from build123d import *

# Parameters (mm, degrees)
SKETCH1_W                                  = 43
SKETCH1_H                                  = 43
SKETCH1_R                                  = 1
BOSS_EXTRUDE1_DEPTH                        = 3.5
SKETCH3_R                                  = 1.45
BOSS_EXTRUDE2_DEPTH                        = 5
MIRROR2_AT_THE_SECOND_PLANE_COPY_1_SKETC_R = 1.45
MIRROR2_AT_THE_SECOND_PLANE_COPY_1_DEPTH   = 5
SKETCH4_W                                  = 4.5
SKETCH4_H                                  = 43
BOSS_EXTRUDE3_DEPTH                        = 5.03


with BuildPart() as part:
    # Sketch1 → Boss-Extrude1 (new body)
    with BuildSketch(Plane(origin=(0, 0, 0), x_dir=(1, 0, 0), z_dir=(0, 1, 0))):
        Rectangle(SKETCH1_W, SKETCH1_H)
        with Locations(Location((0, 0, 0), (0, 0, 270))):
            Circle(SKETCH1_R, mode=Mode.SUBTRACT)
    extrude(amount=BOSS_EXTRUDE1_DEPTH)

    # Sketch3 → Boss-Extrude2 (add)
    with BuildSketch(Plane(origin=(0, 3.5, 0), x_dir=(1, 0, 0), z_dir=(0, 1, 0))):
        with Locations(Location((-18.5, 18.527041475, 0), (0, 0, 90))):
            Circle(SKETCH3_R)
    boss_extrude2 = extrude(amount=BOSS_EXTRUDE2_DEPTH)

    # Mirror2: Boss-Extrude2 across plane
    add(boss_extrude2.mirror(Plane.XY))

    # Mirror2 at the second plane: Boss-Extrude2 across plane
    add(boss_extrude2.mirror(Plane(origin=(0, 0, 0), x_dir=(0, 0, 1), z_dir=(1, 0, 0))))

    # Mirror2 at the second plane copy 1 sketc → Mirror2 at the second plane copy 1 (add)
    with BuildSketch(Plane(origin=(0, 3.5, 0), x_dir=(-1, 0, 0), z_dir=(0, 1, 0))):
        with Locations(Location((-18.5, 18.527041475, 0), (0, 0, 90))):
            Circle(MIRROR2_AT_THE_SECOND_PLANE_COPY_1_SKETC_R)
    extrude(amount=MIRROR2_AT_THE_SECOND_PLANE_COPY_1_DEPTH)

    # Sketch4 → Boss-Extrude3 (add)
    with BuildSketch(Plane.XZ):
        with Locations((-6.625, 0)):
            Rectangle(SKETCH4_W, SKETCH4_H)
    boss_extrude3 = extrude(amount=BOSS_EXTRUDE3_DEPTH)

    # Mirror3: Boss-Extrude3 across plane
    add(boss_extrude3.mirror(Plane(origin=(0, 0, 0), x_dir=(0, 0, 1), z_dir=(1, 0, 0))))


solid = part.part
CAD build for the part. Positions are in the model's coordinates, mm. A direction names the side the tool comes from. Round coordinates to 2 decimals unless told otherwise and drop trailing zeros. Loops run counter-clockwise (first coordinate to the right, second up) from the corner with the lowest first, then second, coordinate; pieces in that order, holes last.
(1) Cut at C-C (z = -11.5). Give the cut face in (x, y) (3 decimals), plus the area to 3 significant figures.
(2) Wall check: line 1 along X through (y, z) = (0.7, 0); line 2 along X through (y, z) = (-4.5, -9) (3 decimals); line 3 along Y through (x, z) = (7, 14.5). Give the ranges that are in metal, low to high.
(3) Which spindle directions (+Z, -Z, +X, -X, +Y, -Y) get a long thin tool onto all of the face, cutting with end or side? Do faces 5 (the flat face through (-2, 0, 0)), 6 (the cylindrical face through (-17.618, 5.965, -17.376)), 7 (the flat face through (15, 0, 0)), 8 (the flat face through (-15, 0, 0)). Say none if no direction does.
(4) Drop flat-ended pins along their axis: pin 1 (2.5 mm diameter, centred on y = -2, z = 7.5, fed in from -X) (3 decimals); pin 2 (21.5 mm diameter, centred on x = -4.5, z = 9, fed in from +Y); pin 3 (1.5 mm diameter, centred on y = -2, z = 5.5, fed in from +X) (3 decimals). Give the stop position or say it passes through.
(5) Cut at A-A (x = 0). Give the cut face in (y, z).
(6) Two-plate mould, pull along Z, no slides. Class faces 1 (the cylindrical face through (-1, 2, 0)), 2 (the flat face through (0, 1, -21.5)), 3 (the flat face through (-21.5, 2, 0)), 4 (the cylindrical face through (-17.618, 5.965, 17.376)): +Z half, -Z half, draft (parallel to the pull), parting line (faces both ways), or undercut.
(7) Cut at B-B (z = 0). Give the cut face in (x, y) (3 decimals).
(8) Cut at D-D (x = 18.5). Give the cut face in (y, z), plus the area to 4 significant figures.
Findings below:
1. outline: (-21.5, 0) - (-8.875, 0) - (-8.875, -5.03) - (-4.375, -5.03) - (-4.375, 0) - (4.375, 0) - (4.375, -5.03) - (8.875, -5.03) - (8.875, 0) - (21.5, 0) - (21.5, 3.5) - (-21.5, 3.5) - close
1. area: 196 mm2
2. line 1: x = -21.5 to -1, 1 to 21.5
2. line 2: x = -8.875 to -4.375, 4.375 to 8.875
2. line 3: y = -5.03 to 3.5
3. face 5: +Z, -Z, -Y
3. face 6: +Y
3. face 7: +Z, -Z, +X, -Y
3. face 8: +Z, -Z, -X, -Y
4. pin 1: stops at x = -8.875
4. pin 2: stops at y = 3.5
4. pin 3: stops at x = 8.875
5. outline: (0, -21.5) - (3.5, -21.5) - (3.5, -1) - (0, -1) - close; (0, 1) - (3.5, 1) - (3.5, 21.5) - (0, 21.5) - close
6. face 1: undercut
6. face 2: -Z half
6. face 3: draft
6. face 4: undercut
7. outline: (-21.5, 0) - (-8.875, 0) - (-8.875, -5.03) - (-4.375, -5.03) - (-4.375, 0) - (-1, 0) - (-1, 3.5) - (-21.5, 3.5) - close; (1, 0) - (4.375, 0) - (4.375, -5.03) - (8.875, -5.03) - (8.875, 0) - (21.5, 0) - (21.5, 3.5) - (1, 3.5) - close
8. outline: (0, -21.5) - (3.5, -21.5) - (3.5, -19.98) - (8.5, -19.98) - (8.5, -17.08) - (3.5, -17.08) - (3.5, 17.08) - (8.5, 17.08) - (8.5, 19.98) - (3.5, 19.98) - (3.5, 21.5) - (0, 21.5) - close
8. area: 179.5 mm2
